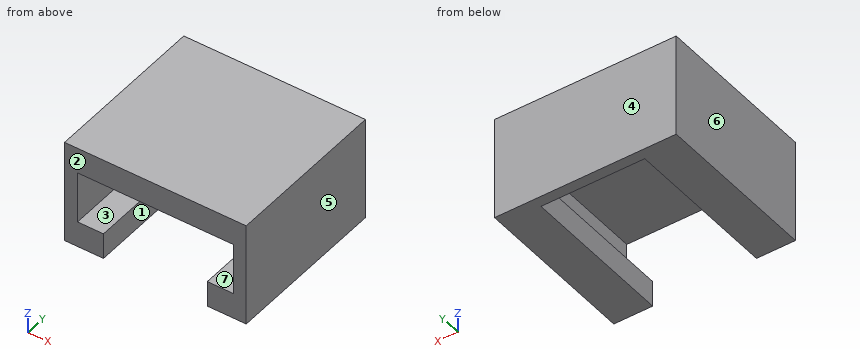
from build123d import *

# Parameters (mm, degrees)
F1_DEPTH      = 75
F1_DEPTH_BACK = 75
F2_W          = 175
F2_H          = 100
F3_DEPTH      = 10


with BuildPart() as f1:
    # F0 (on Front) → F1 (new body, two sides)
    with BuildSketch(Plane.XZ) as f1_sk:
        Polygon((87.5, -50), (87.5, 50), (-87.5, 50), (-87.5, -50), (-50, -50), (-50, -25), (-75, -25), (-75, 25), (75, 25), (75, -25), (50, -25), (50, -50), align=None)
    extrude(amount=F1_DEPTH)
    extrude(f1_sk.sketch, amount=-F1_DEPTH_BACK)

    # F2 (on face) → F3 (join)
    with BuildSketch(Plane(origin=(0, 75, 0), x_dir=(-1, 0, 0), z_dir=(0, 1, 0))):
        Rectangle(F2_W, F2_H)
    extrude(amount=F3_DEPTH)


solid = f1.part
Model file for the job. Use its own axes, mm. Face numbers are marked on the shaded views. A direction names the side the tool comes from. Give positions to 0.01 mm unless a question says otherwise; leave off trailing zeros. Loops run counter-clockwise (first coordinate to the right, second up) from the corner with the lowest first, then second, coordinate; pieces in that order, holes last.
1) Saw through at A-A (x = -72). Write the cut outline in (y, z), plus the area to 3 significant figures.
2) Saw through at C-C (y = 34.5). Write the cut outline in (x, z), plus the area to 3 significant figures.
3) Tool access for the marked faces 1, 2 and 3: list every direction of +Z, -Z, +X, -X, +Y, -Y with a clear straight run to the whole face (end or side of a thin tool).
4) Wall check: line 1 (X direction, y = -32, z = -11); line 2 (Z direction, x = -52.5, y = -39); line 3 (X direction, y = -38, z = -30.5). Give the ranges that are in metal, low to high.
5) Saw through at D-D (x = -20). Write the cut outline in (y, z), plus the area to 3 significant figures.
6) Pull direction X, two halves, no side cores. Call the marked faces 4, 5, 6 and 7: +X half, -X half, draft (parallel to the pull), parting line (faces both ways), or undercut.
7) Flat gauge pins, fed straight in: pin 1 Ø3 at (x, z) = (-34.5, -0.5) entering from -Y; pin 2 Ø5 at (x, y) = (-46, 62.5) entering from -Z; pin 3 Ø12 at (x, z) = (-44.5, 24.5) entering from -Y. Where does each tip first touch, or does it go through?
8) Saw through at B-B (z = -43). Write the cut outline in (x, y), plus the area to 3 significant figures.
Answer block:
1. outline: (-75, -50) - (85, -50) - (85, 50) - (-75, 50) - (-75, 25) - (75, 25) - (75, -25) - (-75, -25) - close
1. area: 8,500 mm2
2. outline: (-87.5, -50) - (-50, -50) - (-50, -25) - (-75, -25) - (-75, 25) - (75, 25) - (75, -25) - (50, -25) - (50, -50) - (87.5, -50) - (87.5, 50) - (-87.5, 50) - close
2. area: 7,500 mm2
3. face 1: -Z, -Y
3. face 2: +Z, -Z, +X, -X, -Y
3. face 3: -Y
4. line 1: x = -87.5 to -75, 75 to 87.5
4. line 2: z = -50 to -25, 25 to 50
4. line 3: x = -87.5 to -50, 50 to 87.5
5. outline: (-75, 25) - (75, 25) - (75, -50) - (85, -50) - (85, 50) - (-75, 50) - close
5. area: 4,750 mm2
6. face 4: draft
6. face 5: +X half
6. face 6: -X half
6. face 7: undercut
7. pin 1: stops at y = 75
7. pin 2: stops at z = 25
7. pin 3: stops at y = -75
8. outline: (-87.5, -75) - (-50, -75) - (-50, 75) - (50, 75) - (50, -75) - (87.5, -75) - (87.5, 85) - (-87.5, 85) - close
8. area: 13,000 mm2
